Work out the finished part from the listing and answer in its coordinate system (mm). Face numbers are marked on the shaded views. A direction names the side the tool comes from. Coordinates: 2 decimals unless noted, no trailing zeros. Write each loop counter-clockwise with the first axis right and the second up, starting at its lowest first coordinate (ties: lowest second). Pieces come first, ordered by that corner, then holes. Notation, with made-up numbers: (46.25, 14) - (99.25, 14) arc R20 cw to (99.25, 22) - close; hole circle Ø1 at (-10, -4.5). An arc over 180 degrees is marked (long way). Use a Markdown table: item, result. Add a question column.
(1) Find the intervals of material crossed by line 1 (Z direction, x = 30.5, y = 24) (3 decimals); line 2 (Y direction, x = 35, z = -22) (3 decimals), in increasing order. Write a range as from..to.
(2) The part is cut by section D-D, the plane y = 16.5. Give the vertices of the cut face in (x, z) (3 decimals).
(3) The part is cut by section C-C, the plane z = -7. Give the vertices of the cut face in (x, y) (1 decimal).
(4) Given pin 1 Ø10.5 at (x, z) = (20, -18) entering from +Y (3 decimals); pin 2 Ø4.5 at (x, y) = (27.559, 15.875) entering from -Z (3 decimals); pin 3 Ø6 at (y, z) = (15, -4) entering from +X, each flat-ended and moving along its own axis, determine where each tip first touches the part or whether it passes through.
(5) The part is cut by section A-A, the plane x = 35. Give the vertices of the cut face in (y, z) (3 decimals).
(6) A tool of negligible diameter and unlimited length cuts with its end or side. For the marked faces 1 and 2, from which of +Z, -Z, +X, -X, +Y, -Y can it reach the whole face along a straight path? Write none if from no direction.
(7) The part is cut by section B-B, the plane x = 19.05. Give the vertices of the cut face in (y, z) (3 decimals).
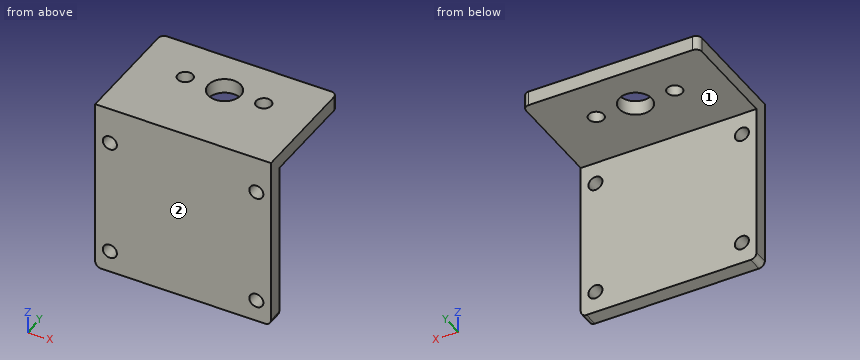
from build123d import *

# Parameters (mm, degrees)
BOSS_EXTRUDE1_DEPTH = 38.1
SKETCH3_R           = 3.5179
SKETCH3_R_2         = 1.6383
CUT_EXTRUDE1_DEPTH  = 4.175
FILLET1_R           = 1.27
SKETCH4_R           = 1.524
CUT_EXTRUDE2_DEPTH  = 4.175


with BuildPart() as part:
    # Sketch2 → Boss-Extrude1 (new body)
    with BuildSketch(Plane(origin=(0, 0, 0), x_dir=(0, 0, -1), z_dir=(1, 0, 0))):
        Polygon((0, 0), (38.1, 0), (38.1, 3.175), (3.175, 3.175), (3.175, 25.4), (0, 25.4), align=None)
    extrude(amount=BOSS_EXTRUDE1_DEPTH)

    # Sketch3 → Cut-Extrude1 (cut, through all)
    with BuildSketch(Plane(origin=(0, 0, -3.175), x_dir=(-1, 0, 0), z_dir=(0, 0, -1))):
        with Locations((-19.05, 15.875)):
            Circle(SKETCH3_R)
        with Locations((-10.541, 15.875)):
            Circle(SKETCH3_R_2)
        with Locations((-27.559, 15.875)):
            Circle(SKETCH3_R_2)
    extrude(amount=-CUT_EXTRUDE1_DEPTH, mode=Mode.SUBTRACT)

    # Fillet1
    fillet1_edges = [part.edges().sort_by_distance(p)[0] for p in [
        (38.1, 1.5875, -38.1),
        (38.1, 25.4, -1.5875),
        (0, 25.4, -1.5875),
        (0, 1.5875, -38.1),
    ]]
    fillet(fillet1_edges, radius=FILLET1_R)

    # Sketch4 → Cut-Extrude2 (cut, through all)
    with BuildSketch(Plane(origin=(0, 3.175, 0), x_dir=(1, 0, 0), z_dir=(0, 1, 0))):
        with Locations((3.175, 7.9502)):
            Circle(SKETCH4_R)
        with Locations((3.175, 33.3502)):
            Circle(SKETCH4_R)
        with Locations((34.925, 33.3502)):
            Circle(SKETCH4_R)
        with Locations((34.925, 7.9502)):
            Circle(SKETCH4_R)
    extrude(amount=-CUT_EXTRUDE2_DEPTH, mode=Mode.SUBTRACT)


solid = part.part
Model answer:
| question | item | result |
|---|---|---|
| 1 | line 1 | -3.175..0 |
| 1 | line 2 | 0..3.175 |
| 2 | outline | (0, -3.175) - (9.027, -3.175) - (9.027, 0) - (0, 0) - close; (12.055, -3.175) - (15.588, -3.175) - (15.588, 0) - (12.055, 0) - close; (22.512, -3.175) - (26.045, -3.175) - (26.045, 0) - (22.512, 0) - close; (29.073, -3.175) - (38.1, -3.175) - (38.1, 0) - (29.073, 0) - close |
| 3 | outline | (0, 0) - (2, 0) - (2, 3.2) - (0, 3.2) - close; (4.4, 0) - (33.7, 0) - (33.7, 3.2) - (4.4, 3.2) - close; (36.1, 0) - (38.1, 0) - (38.1, 3.2) - (36.1, 3.2) - close |
| 4 | pin 1 | y = 3.175 |
| 4 | pin 2 | z = -3.175 |
| 4 | pin 3 | x = 38.1 |
| 5 | outline | (0, -38.1) - (3.175, -38.1) - (3.175, -34.872) - (0, -34.872) - close; (0, -31.828) - (3.175, -31.828) - (3.175, -9.472) - (0, -9.472) - close; (0, -6.428) - (3.175, -6.428) - (3.175, -3.175) - (25.4, -3.175) - (25.4, 0) - (0, 0) - close |
| 6 | face 1 | -Z, +X, -X, +Y |
| 6 | face 2 | +Z, -Z, +X, -X, -Y |
| 7 | outline | (0, -38.1) - (3.175, -38.1) - (3.175, -3.175) - (12.357, -3.175) - (12.357, 0) - (0, 0) - close; (19.393, -3.175) - (25.4, -3.175) - (25.4, 0) - (19.393, 0) - close |
